Geometry check sheet. Reference: the model listing, model coordinates, mm. A direction names the side the tool comes from. Coordinates: 2 decimals unless noted, no trailing zeros. Loops run counter-clockwise (first coordinate to the right, second up) from the corner with the lowest first, then second, coordinate; pieces in that order, holes last.
from build123d import *

# Parameters (mm, degrees)
F0_W     = 25.4
F0_H     = 19.05
F1_DEPTH = 9.525
F2_W     = 15.2418981306
F2_H     = 19.05
F3_DEPTH = 19.05


# Not quite as in the source:
# - a feature names something its author has since deleted; it is built from what else it names


with BuildPart() as f1:
    # F0 (on Right) → F1 (new body, symmetric)
    with BuildSketch(Plane.YZ):
        with Locations((-12.7, 9.525)):
            Rectangle(F0_W, F0_H)
    extrude(amount=F1_DEPTH, both=True)

    # F2 (on face) → F3 (cut)
    with BuildSketch(Plane.XZ.offset(25.4)):
        with Locations((-0.004085945, 9.525)):
            Rectangle(F2_W, F2_H)
    extrude(amount=-F3_DEPTH, mode=Mode.SUBTRACT)


solid = f1.part
(1) Scan lines: L1, parallel to X at y = -16, z = 17 (3 decimals); L2, parallel to Y at x = -0.5, z = 12.5. Record each from-to range of solid material in increasing order.
Findings:
L1: x = -9.525 to -7.625, 7.617 to 9.525
L2: y = -6.35 to 0
(2) Access from +Z, -Z, +X, -X, +Y, -Y to the whole of each face (thin tool, end or side, straight path). Record for faces 1 (the flat face through (0, 0, 9)), 2 (the flat face through (0, -6.35, 10)).
Findings:
face 1: +Z, -Z, +X, -X, +Y
face 2: +Z, -Z, -Y
(3) Draft check along X on faces 3 (the flat face through (7.617, -16, 9)), 4 (the flat face through (-9.525, -13, 10)), 5 (the flat face through (9.525, -13, 10)), 6 (the flat face through (-7.625, -16, 9)). Enter one of: +X half, -X half, draft (parallel to the pull), parting line (faces both ways), or undercut.
Findings:
face 3: undercut
face 4: -X half
face 5: +X half
face 6: undercut
(4) Sectioned sample at B-B on z = 4.75. Record the cut outline in (x, y) (3 decimals), and give its area (3 significant figures).
Findings:
outline: (-9.525, -25.4) - (-7.625, -25.4) - (-7.625, -6.35) - (7.617, -6.35) - (7.617, -25.4) - (9.525, -25.4) - (9.525, 0) - (-9.525, 0) - close
area: 194 mm2
(5) Sectioned sample at A-A on y = -14. Record the cut outline in (x, z) (3 decimals).
Findings:
outline: (-9.525, 0) - (-7.625, 0) - (-7.625, 19.05) - (-9.525, 19.05) - close; (7.617, 0) - (9.525, 0) - (9.525, 19.05) - (7.617, 19.05) - close
(6) Sectioned sample at C-C on x = 3.5. Record the cut outline in (y, z).
Findings:
outline: (-6.35, 0) - (0, 0) - (0, 19.05) - (-6.35, 19.05) - close
